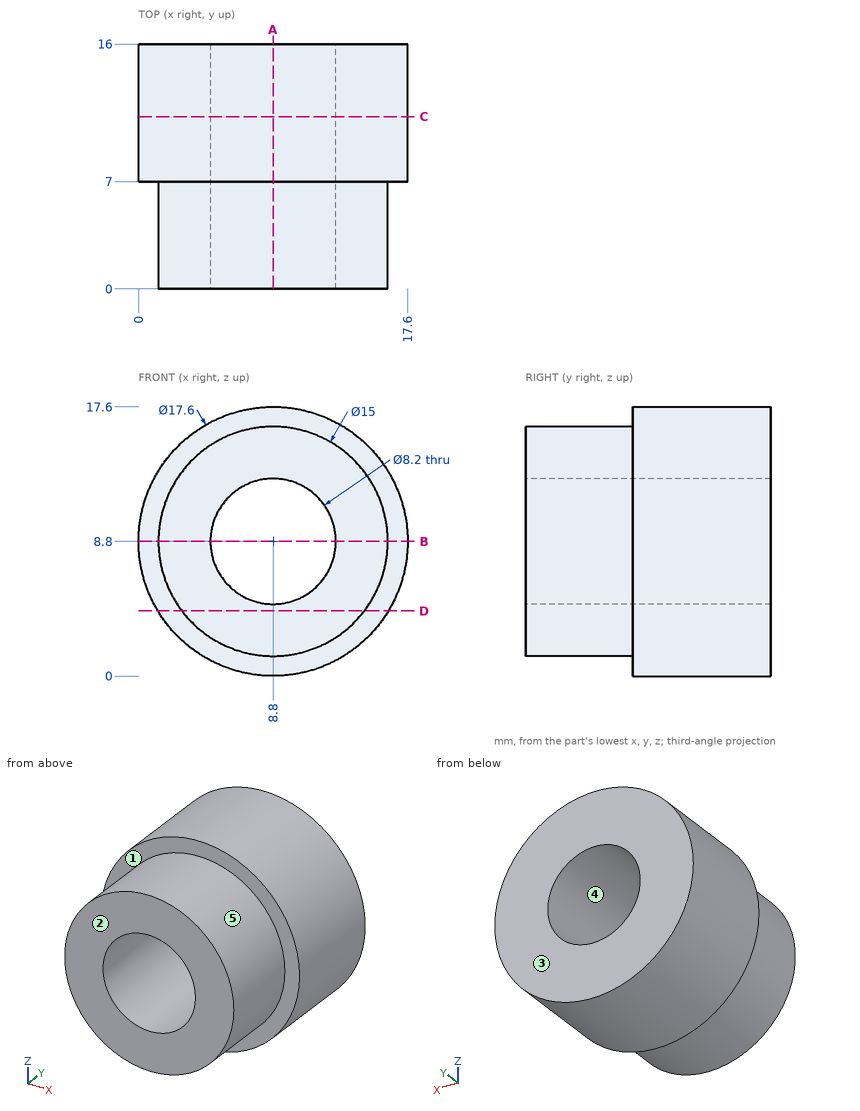
Part print with two shaded views. Sizes in mm from the minimum x, y, z corner. A direction names the side the tool comes from. Give positions to 0.01 mm unless a question says otherwise; leave off trailing zeros. Order: outer loops, then holes, each group sorted by start corner. A loop starts at its lowest first (then second) coordinate and runs counter-clockwise, first axis right, second up.
1) Wall check: probe 1 along Z at (x, y) = (8.8, 8.25); probe 2 along Z at (x, y) = (8.8, 6.5); probe 3 along X at (y, z) = (10.25, 10.25). Give the ranges that are in metal, low to high.
2) Mould opens along X. For the marked faces 3, 4 and 5 say: +X half, -X half, draft (parallel to the pull), parting line (faces both ways), or undercut.
3) Saw through at C-C, the plane y = 11.25. Write the cut outline in (x, z).
4) Pin check, flat tips, straight feed: pin 1 (4 mm diameter, centred on x = 13, y = 5.5, fed in from -Z); pin 2 (3 mm diameter, centred on y = 2, z = 13, fed in from -X); pin 3 (1 mm diameter, centred on y = 11, z = 8, fed in from +X). Stop position of each tip, or through.
5) Saw through at A-A, the plane x = 8.8. Write the cut outline in (y, z).
6) Saw through at D-D, the plane z = 4.25. Write the cut outline in (x, y).
7) 3-axis set-ups, long thin cutter, end or side, ignore diameter. For the marked faces 1 and 2: which of +Z, -Z, +X, -X, +Y, -Y reach the whole face in a straight line?
8) Saw through at B-B, the plane z = 8.8. Write the cut outline in (x, y).
Computed:
1. probe 1: z = 0 to 4.7, 12.9 to 17.6
1. probe 2: z = 1.3 to 4.7, 12.9 to 16.3
1. probe 3: x = 0.12 to 4.96, 12.64 to 17.48
2. face 3: draft
2. face 4: undercut
2. face 5: parting line
3. outline: circle Ø17.6 at (8.8, 8.8); hole circle Ø8.2 at (8.8, 8.8)
4. pin 1: stops at z = 0.48
4. pin 2: stops at x = 1.8
4. pin 3: stops at x = 17.59
5. outline: (0, 1.3) - (7, 1.3) - (7, 0) - (16, 0) - (16, 4.7) - (0, 4.7) - close; (0, 12.9) - (16, 12.9) - (16, 17.6) - (7, 17.6) - (7, 16.3) - (0, 16.3) - close
6. outline: (1.27, 7) - (2.84, 7) - (2.84, 0) - (14.76, 0) - (14.76, 7) - (16.33, 7) - (16.33, 16) - (1.27, 16) - close
7. face 1: -Y
7. face 2: +Z, -Z, +X, -X, -Y
8. outline: (0, 7) - (1.3, 7) - (1.3, 0) - (4.7, 0) - (4.7, 16) - (0, 16) - close; (12.9, 0) - (16.3, 0) - (16.3, 7) - (17.6, 7) - (17.6, 16) - (12.9, 16) - close
